from build123d import *

# Parameters (mm, degrees)
F1_DEPTH = 12.7
F2_R     = 6.35
F3_DEPTH = 25.401
F4_R     = 5.08


with BuildPart() as f1:
    # F0 (on Front) → F1 (new body, symmetric)
    with BuildSketch(Plane.XZ):
        with BuildLine():
            Line((50.8, 25.4), (-50.8, 25.4))
            Line((-50.8, 25.4), (-50.8, -50.8))
            Line((-50.8, -50.8), (-25.4, -50.8))
            Line((-25.4, -50.8), (-25.4, -12.7))
            ThreePointArc((-25.4, -12.7), (-21.680256, -3.719744), (-12.7, 0))
            Line((-12.7, 0), (50.8, 0))
            Line((50.8, 0), (50.8, 25.4))
        make_face()
    extrude(amount=F1_DEPTH, both=True)

    # F2 (on face) → F3 (cut, through all)
    with BuildSketch(Plane.XZ.offset(12.7)):
        with Locations((-31.75, 12.7)):
            Circle(F2_R)
        with Locations((31.75, 12.7)):
            Circle(F2_R)
    extrude(amount=-F3_DEPTH, mode=Mode.SUBTRACT)

    # F4
    f4_edges = [f1.edges().sort_by_distance(p)[0] for p in [
        (50.8, 0, 25.4),
        (50.8, 0, 0),
        (-25.4, 0, -50.8),
        (-50.8, 0, 25.4),
        (-50.8, 0, -50.8),
    ]]
    fillet(f4_edges, radius=F4_R)


solid = f1.part
Input: part model. Units: mm. Frame: model coordinates. A direction names the side the tool comes from. Give positions to 0.01 mm unless a question says otherwise; leave off trailing zeros. Order: outer loops, then holes, each group sorted by start corner. A loop starts at its lowest first (then second) coordinate and runs counter-clockwise, first axis right, second up. Notation, with made-up numbers: M 63,-12.5 L 89,-12.5 A20 cw 89,26.5 Z; hole C -34,3 d8. An arc over 180 degrees is marked long. Answer as a JSON object with one key per item and string values.
1. Cut plane B-B, the plane y = -2. Output: boundary loops of the cut face in (x, z), and give its area (3 significant figures).
Result sheet:
{"outline": "M -50.8,-45.72 A5.08 ccw -45.72,-50.8 L -30.48,-50.8 A5.08 ccw -25.4,-45.72 L -25.4,-12.7 A12.7 cw -12.7,0 L 45.72,0 A5.08 ccw 50.8,5.08 L 50.8,20.32 A5.08 ccw 45.72,25.4 L -45.72,25.4 A5.08 ccw -50.8,20.32 Z; hole C -31.75,12.7 d12.7; hole C 31.75,12.7 d12.7", "area": "3,620 mm²"}
2. Cut plane D-D, the plane x = 31.75. Output: boundary loops of the cut face in (y, z).
Result sheet:
{"outline": "M -12.7,0 L 12.7,0 L 12.7,6.35 L -12.7,6.35 Z; M -12.7,19.05 L 12.7,19.05 L 12.7,25.4 L -12.7,25.4 Z"}
3. Cut plane A-A, the plane x = -31.75. Output: boundary loops of the cut face in (y, z), and give its area (3 significant figures).
Result sheet:
{"outline": "M -12.7,-50.8 L 12.7,-50.8 L 12.7,6.35 L -12.7,6.35 Z; M -12.7,19.05 L 12.7,19.05 L 12.7,25.4 L -12.7,25.4 Z", "area": "1,610 mm²"}
4. Reachability of faces 4 (the flat face through (-25.4, 0, -29)), 5 (the flat face through (1, 0, 25.4)) from +Z, -Z, +X, -X, +Y, -Y: full face, straight path, thin tool, end or side. Return the list, or none.
Result sheet:
{"face 4": "-Z, +X, +Y, -Y", "face 5": "+Z, +X, -X, +Y, -Y"}
5. First-contact query: P1, Ø7.5, axis at y = -4, z = -26.5, coming from the +X side; P2, Ø10, axis at x = 33, y = -7.5, coming from the -Z side; P3, Ø1.5, axis at x = -13, z = -2.5, coming from the -Y side. Flat tips, straight axial feed; report the tip coordinate or a pass-through.
Result sheet:
{"P1": "x = -25.4", "P2": "z = 0", "P3": "through"}
6. Ray query, line 1 (X direction, y = -10.25, z = 11); line 2 (Z direction, x = -31.75, y = -6); line 3 (X direction, y = 6.75, z = -30.5). Return the intervals inside material, ascending. Write a range as [from, to].
Result sheet:
{"line 1": "[-50.8, -37.87], [-25.63, 25.63], [37.87, 50.8]", "line 2": "[-50.8, 6.35], [19.05, 25.4]", "line 3": "[-50.8, -25.4]"}
7. Pull-direction query (X, two-part tool) for faces 1 (the cylindrical face through (35.164, -0.178, 18.054)), 2 (the cylindrical face through (-21.78, -0.18, -3.82)), 3 (the flat face through (16, 0, 0)); classes: +X half, -X half, draft (parallel to the pull), parting line (faces both ways), or undercut.
Result sheet:
{"face 1": "undercut", "face 2": "+X half", "face 3": "draft"}
8. Cut plane C-C, the plane z = 12.7. Output: boundary loops of the cut face in (x, y), and give its area (3 significant figures).
Result sheet:
{"outline": "M -50.8,-12.7 L -38.1,-12.7 L -38.1,12.7 L -50.8,12.7 Z; M -25.4,-12.7 L 25.4,-12.7 L 25.4,12.7 L -25.4,12.7 Z; M 38.1,-12.7 L 50.8,-12.7 L 50.8,12.7 L 38.1,12.7 Z", "area": "1,940 mm²"}
